Autodesk Inventor part; units mm, degrees
ref_plane "YZ Plane" through (0, 0, 0) normal (1, 0, 0) x (0, 1, 0)
ref_plane "XZ Plane" through (0, 0, 0) normal (0, 1, 0) x (-1, 0, 0)
ref_plane "XY Plane" through (0, 0, 0) normal (0, 0, 1) x (1, 0, 0)
sketch "Sketch1" plane through (0, 0, 0) normal (1, 0, 0) x (0, 1, 0)
  line L0 (-12.7635, 12.7635) -> (12.7635, 12.7635)
  line L1 (12.7635, 12.7635) -> (12.7635, -12.7635)
  line L2 (12.7635, -12.7635) -> (-12.7635, -12.7635)
  line L3 (-12.7635, -12.7635) -> (-12.7635, 12.7635)
  line L4 (-12.7635, 12.7635) -> (12.7635, -12.7635) construction
  line L5 (12.7635, 12.7635) -> (-12.7635, -12.7635) construction
  line L6 (19.1135, 19.1135) -> (-19.1135, 19.1135)
  line L7 (-19.1135, 19.1135) -> (-19.1135, -19.1135)
  line L8 (-19.1135, -19.1135) -> (19.1135, -19.1135)
  line L9 (19.1135, -19.1135) -> (19.1135, 19.1135)
  line L10 (12.7635, 19.1135) -> (12.7635, -19.1135)
  line L11 (-19.1135, -5.4793) -> (-46.5737, -5.4793)
  line L12 (-46.5737, -5.4793) -> (-46.5737, -19.1135)
  line L13 (-46.5737, -19.1135) -> (-19.1135, -19.1135)
  line L14 (-19.1135, -19.1135) -> (-19.1135, -5.4793)
  point P0 (0, 0)
  point P1 (12.7635, 12.7635)
  dimension "d1" = 25.527
  dimension "d2" = 6.35
extrude "Extrusion1" add sketch "Sketch1" along normal blind 50.8 contours L3 L2 L10 L8 L7 L6 L0 | L13 L12 L11 L7
sketch "Sketch2" plane through (0, -46.5737, -5.4793) normal (0, 0, 1) x (1, 0, 0)
  line L0 (0, 27.4602) -> (0, 0)
  line L1 (0, 0) -> (50.8, 0)
  line L2 (50.8, 27.4602) -> (50.8, 0)
  line L3 (0, 27.4602) -> (50.8, 27.4602)
  circle A0 centre (36.2123, 13.7301) radius 7
  point P0 (0, 46.5737)
  dimension "d5" = 14
extrude "Extrusion2" cut sketch "Sketch2" against normal through all contours A0
sketch "Sketch3" plane through (0, -46.5737, -19.1135) normal (0, 0, -1) x (-1, 0, 0)
  circle A0 centre (-36.2123, 13.7301) radius 7
  circle A1 centre (-36.2123, 13.7301) radius 11
  point P0 (0, 46.5737)
  dimension "d8" = 22
extrude "Extrusion3" cut sketch "Sketch3" against normal blind 5
sketch "Sketch4" plane through (0, -12.7635, 12.7635) normal (0, 1, 0) x (1, 0, 0)
  line L0 (0, 25.527) -> (0, 0)
  line L1 (0, 0) -> (50.8, 0)
  line L2 (50.8, 25.527) -> (50.8, 0)
  line L3 (0, 25.527) -> (50.8, 25.527)
  line L4 (0, 12.7635) -> (50.8, 12.7635) construction
  circle A0 centre (9.0739, 12.7635) radius 2.5
  circle A1 centre (25.4, 12.7635) radius 2.5
  circle A2 centre (40.9031, 12.7635) radius 2.5
  dimension "d11" = 5
  dimension "d12" = 5
  dimension "d13" = 5
extrude "Extrusion4" cut sketch "Sketch4" against normal through all contours A0 | A1 | A2
sketch "Sketch5" plane through (0, -12.7635, 12.7635) normal (0, 0, -1) x (-1, 0, 0)
  line L0 (-43.4031, 0) -> (-38.4031, 0)
  line L1 (-27.9, 0) -> (-22.9, 0)
  line L2 (-11.5739, 0) -> (-6.5739, 0)
  line L3 (0, 0) -> (0, 25.527)
  line L4 (0, 25.527) -> (-50.8, 25.527)
  line L5 (-50.8, 0) -> (-50.8, 25.527)
  line L6 (0, 0) -> (-50.8, 0)
  circle A0 centre (-9.0739, 12.7635) radius 2.5
  circle A1 centre (-25.4, 12.7635) radius 2.5
  circle A2 centre (-40.9031, 12.7635) radius 2.5
  point P0 (0, 12.7635)
  dimension "d16" = 5
extrude "Extrusion5" cut sketch "Sketch5" along normal through all both and the other way through all contours A0 | A1 | A2
sketch "Sketch7" plane through (0, -46.5737, -5.4793) normal (0, 0, 1) x (1, 0, 0)
  circle A0 centre (36.2123, 13.7301) radius 7
  circle A1 centre (36.2123, 13.7301) radius 11
  point P0 (0, 46.5737)
  dimension "d21" = 22
extrude "Extrusion7" cut sketch "Sketch7" against normal blind 3
sketch "Sketch8" plane through (0, -46.5737, -5.4793) normal (0, 0, 1) x (1, 0, 0)
  line L0 (0, 27.4602) -> (0, 0)
  circle A0 centre (36.2123, 13.7301) radius 11
  line L1 (0, 27.4602) -> (0, 0)
  line L2 (0, 0) -> (50.8, 0)
  line L3 (50.8, 27.4602) -> (50.8, 0)
  line L4 (0, 27.4602) -> (50.8, 27.4602)
  circle A1 centre (9.5855, 21.0501) radius 2.5
  line L5 (0, 0) -> (0, 59.3372)
  line L6 (0, 14.2925) -> (25.4, 0)
  point P0 (0, 46.5737)
  point P1 (0, 14.2925)
  dimension "d24" = 5
extrude "Extrusion8" cut sketch "Sketch8" along normal through all both and the other way through all contours L6 L2 L0 | A1
fillet "Fillet1" radius 12.7 3 edges at (0, -32.2813, -12.2964) (50.8, -46.5737, -12.2964) (25.4, -46.5737, -12.2964)
sketch "Sketch9" plane through (0, -19.1135, -5.4793) normal (0, 0, 1) x (1, 0, 0)
  circle A0 centre (9.5855, -6.4101) radius 2.5
  circle A1 centre (36.2123, -13.7301) radius 11
  arc A2 (22.4998, -25.8283) -> (28.7278, -27.4602) centre (28.7278, -14.7602) ccw
  line L0 (28.7278, -27.4602) -> (38.1, -27.4602)
  arc A3 (38.1, -27.4602) -> (50.8, -14.7602) centre (38.1, -14.7602) ccw
  line L1 (50.8, 0) -> (50.8, -14.7602)
  line L2 (0, 0) -> (50.8, 0)
  line L3 (0, 0) -> (0, -5.7415)
  arc A4 (0, -5.7415) -> (6.472, -16.8095) centre (12.7, -5.7415) ccw
  line L4 (6.472, -16.8095) -> (22.4998, -25.8283)
  circle A5 centre (9.5855, -6.4101) radius 5.3589
  point P0 (0, 19.1135)
extrude "Extrusion9" cut sketch "Sketch9" against normal blind 5 contours A5
fillet "Fillet2" radius 3.175 1 edges at (25.4, -19.1135, -5.4793)
fillet "Fillet3" radius 3.175 3 edges at (25.4, -19.1135, 19.1135) (25.4, 12.7635, 19.1135) (25.4, 12.7635, -19.1135)
properties part number "swingarmBase"
Design review of the part built by this model. Coordinates are the model's own, in mm. A direction names the side the tool comes from. Give positions to 0.01 mm unless a question says otherwise; leave off trailing zeros. Order: outer loops, then holes, each group sorted by start corner. A loop starts at its lowest first (then second) coordinate and runs counter-clockwise, first axis right, second up. Notation, with made-up numbers: (-24, -15) - (-16, -15) arc R10 ccw to (-16, -3) - close; hole circle Ø9 at (44.25, 59.25). An arc over 180 degrees is marked (long way). Use CSV: the item, a comma, the result in double quotes. Start each with the question number.
Q1. Take a section at A-A (y = 8). State the section outline as (x, z) points.
Q2. For P1, Ø2, axis at x = 27, z = 1, coming from the +Y side; P2, Ø3, axis at x = 10, y = -24, coming from the +Z side; P3, Ø6.5, axis at x = 9.07, y = 0, coming from the +Z side; P4, Ø9, axis at x = 35.5, z = 9.5, coming from the -Y side, all flat-tipped, find the tip position at first contact; note any pin that passes through.
Q3. Draft analysis for pull direction Z (two halves, no side actions). For faces 1 (the face through (25, -12.764, -3)), 2 (the face through (11, -28, -10.479)), 3 (the face through (38.6, -43.58, -16.65)), state which applies: pulls with the +Z half, pulls with the -Z half, needs draft (parallel to the pull), parting line crosses it, or undercut.
Q4. Take a section at C-C (y = 0). Count the separate pieces of the cut face and the enclosed holes in it, and give its area (3 significant figures).
Q5. Machinability: for faces 4 (the face through (25, -19.114, 7)), 5 (the face through (41.29, -42.6, -6.94)), 6 (the face through (23.09, 0.96, -15.89)), 7 (the face through (25, -3, 12.764)), 8 (the face through (25, -3, 19.114)), which of the approach directions +Z, -Z, +X, -X, +Y, -Y give a long, thin tool a straight path to every point of the face, cutting with its end or side? Answer none if there is none.
Q6. For line 1 (X direction, y = -25.5, z = -12); line 2 (X direction, y = 0, z = -17.5); line 3 (Y direction, x = 25.4, z = 15.25), list the stretches that pass through material, from the lowest coordinate up.
Q7. Take a section at B-B (z = 0). State the section outline as (x, y) points, and give its area (3 significant figures).
Calculated:
1,outline,"(0, -19.11) - (50.8, -19.11) - (50.8, -12.76) - (0, -12.76) - close; (0, 12.76) - (50.8, 12.76) - (50.8, 19.11) - (0, 19.11) - close"
2,P1,"stops at y = -12.76"
2,P2,"stops at z = -10.48"
2,P3,"stops at z = 19.11"
2,P4,"stops at y = -19.11"
3,face 1,"undercut"
3,face 2,"pulls with the +Z half"
3,face 3,"needs draft"
4,separate pieces,"8"
4,enclosed holes,"0"
4,area,"455 mm²"
5,face 4,"+Z, +X, -X, -Y"
5,face 5,"+Z"
5,face 6,"+Z, -Z"
5,face 7,"+X, -X, +Y"
5,face 8,"+Z, +X, -X, +Y, -Y"
6,line 1,"x = 0.02 to 7.09, 12.09 to 50.8"
6,line 2,"x = 0 to 6.57, 11.57 to 22.9, 27.9 to 38.4, 43.4 to 50.8"
6,line 3,"y = -19.11 to -2.5, 2.5 to 12.76"
7,outline,"(0, -19.11) - (6.57, -19.11) - (6.57, -12.76) - (0, -12.76) - close; (11.57, -19.11) - (22.9, -19.11) - (22.9, -12.76) - (11.57, -12.76) - close; (27.9, -19.11) - (38.4, -19.11) - (38.4, -12.76) - (27.9, -12.76) - close; (43.4, -19.11) - (50.8, -19.11) - (50.8, -12.76) - (43.4, -12.76) - close"
7,area,"227 mm²"
